The drawing under review shows one solid part. Ordinate dimensions are in mm from its lowest x, y, z. Give positions to 0.01 mm unless a question says otherwise; leave off trailing zeros. Loops run counter-clockwise (first coordinate to the right, second up) from the corner with the lowest first, then second, coordinate; pieces in that order, holes last.
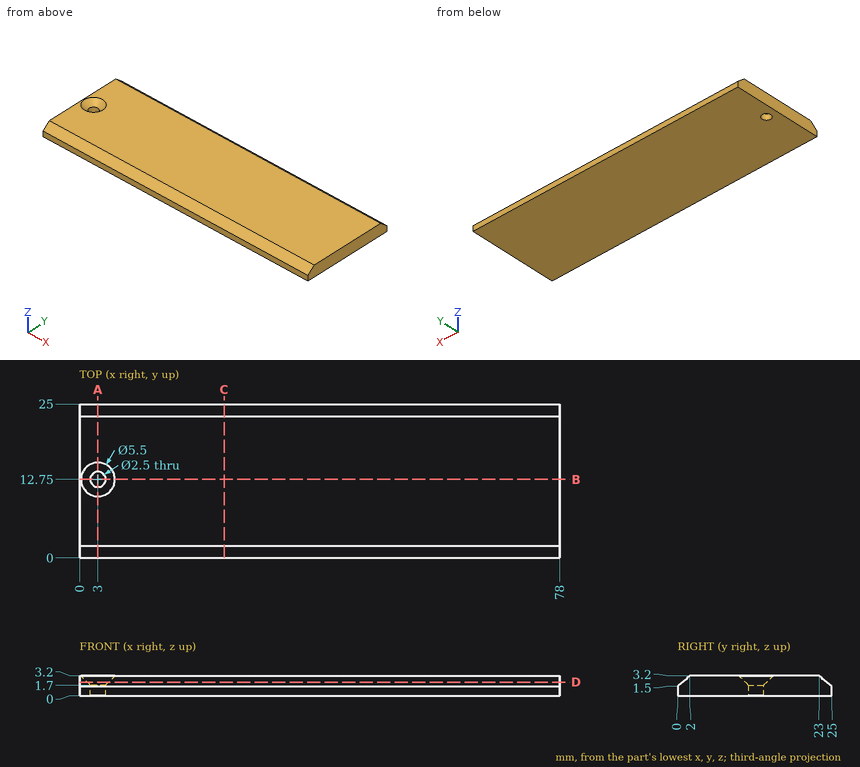
Item 1: Take a section at C-C on x = 23.5. Give the boundary of the cut face in (y, z).
Answer:
outline: (0, 0) - (25, 0) - (25, 1.5) - (23, 3.2) - (2, 3.2) - (0, 1.5) - close
Item 2: Take a section at D-D on z = 2.2. Give the boundary of the cut face in (x, y), and give its area (3 significant figures).
Answer:
outline: (0, 0.82) - (78, 0.82) - (78, 24.18) - (0, 24.18) - close; hole circle Ø3.5 at (3, 12.75)
area: 1,810 mm2
Item 3: For L1, parallel to X at y = 12.75, z = 1.4; L2, parallel to Y at x = 25, z = 2.8; L3, parallel to Y at x = 49.5, z = 2.4, list the stretches that pass through material, from the lowest coordinate up.
Answer:
L1: x = 0 to 1.75, 4.25 to 78
L2: y = 1.53 to 23.47
L3: y = 1.06 to 23.94
Item 4: Clearance check with a flat-ended pin moving along its axis: pin 1 Ø1.5 at (x, y) = (16.5, 20) entering from -Z. State where the tip first meets the part, or that it passes through.
Answer:
pin 1: stops at z = 0
Item 5: Take a section at B-B on y = 12.75. Give the boundary of the cut face in (x, z).
Answer:
outline: (0, 0) - (1.75, 0) - (1.75, 1.7) - (0.25, 3.2) - (0, 3.2) - close; (4.25, 0) - (78, 0) - (78, 3.2) - (5.75, 3.2) - (4.25, 1.7) - close
Item 6: Take a section at A-A on x = 3. Give the boundary of the cut face in (y, z).
Answer:
outline: (0, 0) - (11.5, 0) - (11.5, 1.7) - (10, 3.2) - (2, 3.2) - (0, 1.5) - close; (14, 0) - (25, 0) - (25, 1.5) - (23, 3.2) - (15.5, 3.2) - (14, 1.7) - close
